Read the model definition and answer for the solid it produces. Units are mm, in the model's axes. Coordinates: 2 decimals unless noted, no trailing zeros. Loops run counter-clockwise (first coordinate to the right, second up) from the corner with the lowest first, then second, coordinate; pieces in that order, holes last.
from build123d import *

# Parameters (mm, degrees)
SKETCH1_W            = 157.271841604
SKETCH1_H            = 85.34874331
BOSS_EXTRUDE1_DEPTH  = 25.4
CUT_SWEEP2_PROFILE_R = 5.08


with BuildPart() as part:
    # Sketch1 → Boss-Extrude1 (new, symmetric)
    with BuildSketch(Plane(origin=(0, 0, 0), x_dir=(0, 0, -1), z_dir=(1, 0, 0))):
        Rectangle(SKETCH1_W, SKETCH1_H)
    extrude(amount=BOSS_EXTRUDE1_DEPTH, both=True)

    # Cut-Sweep2: sweep along a path in Sketch11
    with BuildLine(Plane(origin=(0, 0, 0), x_dir=(0, 0, -1), z_dir=(1, 0, 0))) as cut_sweep2_path:
        Line((-86.885944584, 0), (-36.013867587, 0))
        Line((-36.013867587, 0), (-23.506619997, 28.372870033))
        Line((-23.506619997, 28.372870033), (26.452653889, 28.372870033))
        Line((26.452653889, 28.372870033), (46.242947448, 0))
        Line((46.242947448, 0), (78.869898607, 0))
    # Cut-Sweep2 profile (on start of the path) → Cut-Sweep2 (sweep, cut)
    with BuildSketch(Plane(origin=(0, 0, 86.885944584), x_dir=(-1, 0, 0), z_dir=(0, 0, -1))):
        Circle(CUT_SWEEP2_PROFILE_R)
    sweep(path=cut_sweep2_path.line, transition=Transition.RIGHT, mode=Mode.SUBTRACT)


solid = part.part
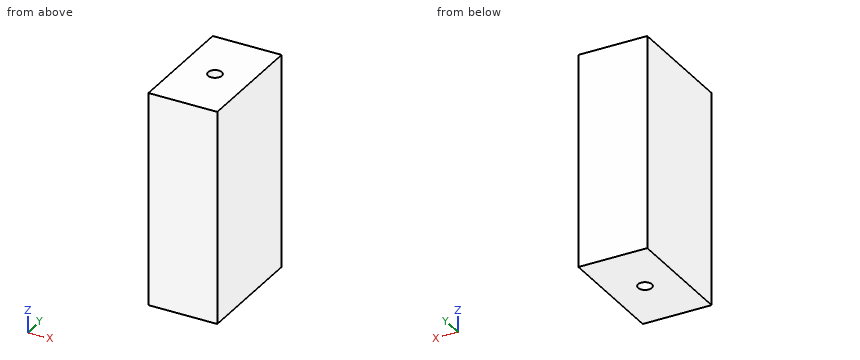
Q1. Straight lines are drawn through the part: probe 1 along X at (y, z) = (0, -67); probe 2 along Y at (x, z) = (0, 64); probe 3 along Z at (x, y) = (-2, 14). For each, find the intervals that lie inside material, in ascending order.
Findings below:
probe 1: x = -25.4 to -5.08, 5.08 to 25.4
probe 2: y = -42.67 to -5.08, 5.08 to 42.67
probe 3: z = -78.64 to -42.17, -30.78 to 24.74, 34.95 to 78.64
Q2. A cutting plane is placed at A-A (x = 0). Give the vertices of the cut face in (y, z).
Findings below:
outline: (-42.67, -78.64) - (-5.08, -78.64) - (-5.08, -43.59) - (23.29, -23.8) - (23.29, 20.19) - (-5.08, 32.7) - (-5.08, 78.64) - (-42.67, 78.64) - close; (5.08, -78.64) - (42.67, -78.64) - (42.67, 78.64) - (5.08, 78.64) - (5.08, 39.33) - (33.45, 26.82) - (33.45, -29.1) - (5.08, -48.89) - close
Q3. A flat-ended cylindrical pin translates along its axis: pin 1 Ø1 at (x, y) = (2.5, 0.5) entering from -Z. Find the tip coordinate at first contact, or state that the pin passes through.
Findings below:
pin 1: stops at z = -41.02
Q4. A cutting plane is placed at C-C (y = 7). Count the separate pieces of the cut face and the enclosed holes in it, then the cut area to 3 significant figures.
Findings below:
separate pieces: 1
enclosed holes: 2
area: 7,800 mm2
Q5. A cutting plane is placed at B-B (z = 65.5). Give the vertices of the cut face in (x, y), then the cut area to 3 significant figures.
Findings below:
outline: (-25.4, -42.67) - (25.4, -42.67) - (25.4, 42.67) - (-25.4, 42.67) - close; hole circle Ø10.16 at (0, 0)
area: 4,250 mm2
